Read the model definition and answer for the solid it produces. Units are mm, in the model's axes. Coordinates: 2 decimals unless noted, no trailing zeros. Write each loop counter-clockwise with the first axis right and the second up, starting at its lowest first coordinate (ties: lowest second). Pieces come first, ordered by that corner, then holes. Notation, with made-up numbers: (-33.5, -39) -> (5.5, -39) arc R22 ccw to (5.5, -11) -> close; hole circle Ø9 at (36, 37). An arc over 180 degrees is marked (long way). One line per item, written item: value. Start each with the question number.
1. Find section B-B, the plane y = 75.41. Write down the section's boundary in (x, z), and give its area (3 significant figures).
2. Find section D-D, the plane z = 4.05. State how many separate pieces and enclosed holes the cut face has, and give its area (3 significant figures).
3. For a pull along X with two mould halves and no side action, classify faces 1 (the cylindrical face through (13.788, 45.89, 2.465)), 2 (the flat face through (2, 55, 5)), 3 (the cylindrical face through (-13.79, 78.2, 2.54)), 4 (the cylindrical face through (-13.59, 53.12, 2.46)) as pulls with the +X half, pulls with the -X half, needs draft (parallel to the pull), parting line crosses it, or undercut.
4. Consider line 1 along Y through (x, z) = (12.57, 2.45); line 2 along Y through (x, z) = (-12.6, 1.8); line 3 along X through (y, z) = (56, 2.25). Determine where each line is inside the solid, lowest interval first.
5. Given P1, Ø1, axis at y = 88, z = 2.5, coming from the +X side; P2, Ø2.5, axis at x = 12.77, y = 16.54, coming from the +Z side; P3, Ø3, axis at x = 8.5, z = 4, coming from the -Y side; P4, Ø3, axis at y = 84, z = 0.5, coming from the +X side, each flat-ended and moving along its own axis, determine where each tip first touches the part or whether it passes through.
6. Find section C-C, the plane y = 10. Write down the section's boundary in (x, z), and give its area (3 significant figures).
7. Find section A-A, the plane x = 0. Write down the section's boundary in (y, z).
```python
from build123d import *

# Parameters (mm, degrees)
RESSALTO_EXTRUS_O1_DEPTH = 5
FILETE3_R                = 10
FILETE4_R                = 10
ESBO_O2_R                = 1.5
CORTE_EXTRUS_O1_DEPTH    = 5
ESBO_O3_R                = 1.5
CORTE_EXTRUS_O2_DEPTH    = 121.092170275
ESBO_O4_R                = 1.5
CORTE_EXTRUS_O3_DEPTH    = 10


with BuildPart() as part:
    # Esboço1 → Ressalto-extrusão1 (new body)
    with BuildSketch(Plane.XY):
        with BuildLine():
            ThreePointArc((-10, 0), (0, -10), (10, 0))
            Line((10, 0), (20, 0))
            ThreePointArc((20, 0), (14.071698091, 40.495175194), (14.829943665, 81.414963086))
            ThreePointArc((14.829943665, 81.414963086), (11.193742071, 116.066691762), (-16.576524471, 95.024435265))
            Line((-16.576524471, 95.024435265), (-16.487894969, 94.437265709))
            Line((-16.487894969, 94.437265709), (-16.369382775, 93.652123615))
            ThreePointArc((-16.369382775, 93.652123615), (-13.756795166, 46.654405302), (-20, 0))
            Line((-20, 0), (-10, 0))
        make_face()
    extrude(amount=RESSALTO_EXTRUS_O1_DEPTH)

    # Filete3
    # the kernel refuses this fillet: 10 mm, written as the material it takes off along each edge
    with BuildSketch(Plane(origin=(20, 0, -29.463728433), x_dir=(-0.20232831186330175, 0.9793177493635794, 0), z_dir=(0, 0, 1))) as filete3_piece_1:
        with BuildLine():
            CenterArc((12.021201201, 9.997221658), FILETE3_R, 181.169168083, 87.480189)
            Line((2.023283119, 9.793177494), (1.823324757, 9.78909661))
            ThreePointArc((1.823324757, 9.78909661), (0.815778009, 4.937054409), (-0.19586355, 0.040465662))
            Line((-0.19586355, 0.040465662), (0.004714197, -0.199944433))
            ThreePointArc((0.004714197, -0.199944433), (5.892745687, -0.130541448), (11.780777177, -0.199944433))
            Line((11.780777177, -0.199944433), (11.785491373, 0))
        make_face()
    extrude(amount=63.927456867, mode=Mode.SUBTRACT)
    with BuildSketch(Plane(origin=(-20, 0, -29.463728433), x_dir=(1, 0, 0), z_dir=(0, 0, 1))) as filete3_piece_2:
        with BuildLine():
            CenterArc((12.222685959, 9.749854723), FILETE3_R, 169.67749742, 87.480189)
            Line((2.384538574, 11.541740887), (2.187775626, 11.57757861))
            ThreePointArc((2.187775626, 11.57757861), (1.06442773, 5.797282674), (-0.194855317, 0.045071116))
            Line((-0.194855317, 0.045071116), (0, -0.2))
            ThreePointArc((0, -0.2), (5, -0.2), (9.955546281, -0.194997094))
            Line((9.955546281, -0.194997094), (10, 0))
        make_face()
    extrude(amount=63.927456867, mode=Mode.SUBTRACT)

    # Filete4
    filete4_edges = [part.edges().sort_by_distance(p)[0] for p in [
        (10, 0, 2.5),
        (-10, 0, 2.5),
    ]]
    fillet(filete4_edges, radius=FILETE4_R)

    # Esboço2 → Corte-extrusão1 (cut)
    with BuildSketch(Plane.XY.offset(5)):
        Circle(ESBO_O2_R)
    extrude(amount=-CORTE_EXTRUS_O1_DEPTH, mode=Mode.SUBTRACT)

    # Esboço3 → Corte-extrusão2 (cut, through all)
    with BuildSketch(Plane.XY.offset(5)):
        with Locations((-12.6, 14.5)):
            Circle(ESBO_O3_R)
        with Locations((-12.6, 24.5)):
            Circle(ESBO_O3_R)
        with Locations((-12.6, 79.11)):
            Circle(ESBO_O3_R)
        with Locations((-12.6, 84.11)):
            Circle(ESBO_O3_R)
    extrude(amount=-CORTE_EXTRUS_O2_DEPTH, mode=Mode.SUBTRACT)

    # Esboço4 → Corte-extrusão3 (cut)
    with BuildSketch(Plane.XY.offset(5)):
        with Locations((12.57, 79.41)):
            Circle(ESBO_O4_R)
        with Locations((12.57, 75.41)):
            Circle(ESBO_O4_R)
        with Locations((12.77, 24.54)):
            Circle(ESBO_O4_R)
        with Locations((12.77, 16.54)):
            Circle(ESBO_O4_R)
    extrude(amount=-CORTE_EXTRUS_O3_DEPTH, mode=Mode.SUBTRACT)


solid = part.part
```
Answer block:
1. outline: (-14.3, 0) -> (11.07, 0) -> (11.07, 5) -> (-14.3, 5) -> close; (14.07, 0) -> (14.3, 0) -> (14.3, 5) -> (14.07, 5) -> close
1. area: 128 mm2
2. separate pieces: 1
2. enclosed holes: 9
2. area: 3,730 mm2
3. face 1: pulls with the +X half
3. face 2: needs draft
3. face 3: undercut
3. face 4: pulls with the -X half
4. line 1: y = 0.89 to 15.05, 18.03 to 23.05, 26.03 to 73.91, 76.91 to 77.91, 80.91 to 115.41
4. line 2: y = 0.91 to 13, 16 to 23, 26 to 77.61, 80.61 to 82.61, 85.61 to 109.92
4. line 3: x = -13.57 to 13.57
5. P1: stops at x = 20.99
5. P2: passes through
5. P3: stops at y = -7.14
5. P4: stops at x = 19.08
6. outline: (-17.77, 0) -> (17.77, 0) -> (17.77, 5) -> (-17.77, 5) -> close
6. area: 178 mm2
7. outline: (-10, 0) -> (-1.5, 0) -> (-1.5, 5) -> (-10, 5) -> close; (1.5, 0) -> (117.45, 0) -> (117.45, 5) -> (1.5, 5) -> close
